The listing builds one solid part. Answer for the finished solid, in the listing's coordinates (mm). A direction names the side the tool comes from. Round coordinates to 2 decimals unless told otherwise and drop trailing zeros. Loops run counter-clockwise (first coordinate to the right, second up) from the corner with the lowest first, then second, coordinate; pieces in that order, holes last. Notation, with made-up numbers: M 60,21 L 107,21 A30 ccw 107,54 Z; hole C 32,17.25 d6. An arc over 180 degrees is marked long. Answer as a JSON object with one key per item and string values.
```python
from build123d import *

# Parameters (mm, degrees)
ESBO_O1_R                  = 19
RESSALTO_EXTRUS_O1_DEPTH   = 7.5
CORTE_EXTRUS_O1_DEPTH      = 28.897132469
CORTE_EXTRUS_O1_DEPTH_BACK = 28.897132469
ESBO_O3_R                  = 13.5
RESSALTO_EXTRUS_O2_DEPTH   = 20
FURO_ROSCADO_DE_M61_D      = 5
FURO_ROSCADO_DE_M51_D      = 4.2
FURO_ROSCADO_DE_M51_DEPTH  = 10
FURO_ROSCADO_DE_M51_TIP    = 1.2618073


with BuildPart() as part:
    # Esboço1 → Ressalto-extrusão1 (new, symmetric)
    with BuildSketch(Plane.XY):
        Circle(ESBO_O1_R)
    extrude(amount=RESSALTO_EXTRUS_O1_DEPTH, both=True)

    # Esboço2 → Corte-extrusão1 (cut, two sides: drawn at the far end of the back side and taken through both)
    with BuildSketch(Plane(origin=(0, 0, 0), x_dir=(1, 0, 0), z_dir=(0, 1, 0)).offset(-CORTE_EXTRUS_O1_DEPTH_BACK)):
        with BuildLine():
            Line((-96.112462059, -41.105261283), (-19, 2.5))
            ThreePointArc((-19, 2.5), (0, 7.5), (19, 2.5))
            Line((19, 2.5), (96.112462059, -41.105261283))
            Line((96.112462059, -41.105261283), (96.112462059, 136.069800352))
            Line((96.112462059, 136.069800352), (-96.112462059, 136.069800352))
            Line((-96.112462059, 136.069800352), (-96.112462059, -41.105261283))
        make_face()
    extrude(amount=CORTE_EXTRUS_O1_DEPTH + CORTE_EXTRUS_O1_DEPTH_BACK, mode=Mode.SUBTRACT)

    # Esboço3 → Ressalto-extrusão2 (add)
    with BuildSketch(Plane.XY.offset(7.5)):
        Circle(ESBO_O3_R)
    extrude(amount=RESSALTO_EXTRUS_O2_DEPTH)

    # Furo roscado de M61 (through all)
    with Locations(Plane.XY.offset(27.5)):
        with Locations((0, 0)):
            Hole(FURO_ROSCADO_DE_M61_D / 2)

    # Furo roscado de M51
    with Locations(Plane(origin=(0, 14, 0), x_dir=(1, 0, 0), z_dir=(0, 1, 0))):
        with Locations((0, -17.5)):
            Hole(FURO_ROSCADO_DE_M51_D / 2, depth=FURO_ROSCADO_DE_M51_DEPTH)
            with Locations((0, 0, -(FURO_ROSCADO_DE_M51_DEPTH + FURO_ROSCADO_DE_M51_TIP / 2))):  # 118° drill point
                Cone(0, FURO_ROSCADO_DE_M51_D / 2, FURO_ROSCADO_DE_M51_TIP, mode=Mode.SUBTRACT)


solid = part.part
```
Item 1: The part is cut by section D-D (x = -7). Give the vertices of the cut face in (y, z).
Values follow:
{"outline": "M -17.66,-6.86 L 17.66,-6.86 L 17.66,7.5 L 11.54,7.5 L 11.54,27.5 L -11.54,27.5 L -11.54,7.5 L -17.66,7.5 Z"}
Item 2: Flat-ended cylindrical pins translate along their axes: P1, Ø6.5, axis at x = 0, z = 17.5, coming from the -Y side; P2, Ø3, axis at x = 0, y = 0, coming from the +Z side; P3, Ø1, axis at y = -5.5, z = 9, coming from the +X side; P4, Ø2, axis at x = 12.5, z = 3.5, coming from the +Y side. Find the tip coordinate at first contact, or state that the pin passes through.
Values follow:
{"P1": "y = -13.5", "P2": "through", "P3": "x = 12.54", "P4": "y = 15.12"}
Item 3: Straight lines are drawn through the part: line 1 (Y direction, x = 0, z = 2); line 2 (Y direction, x = 0, z = 14); line 3 (Z direction, x = 0, y = 8.25). For each, find the intervals that lie inside material, in ascending order.
Values follow:
{"line 1": "-19 to -2.5, 2.5 to 19", "line 2": "-13.5 to -2.5, 2.5 to 13.5", "line 3": "-7.5 to 15.4, 19.6 to 27.5"}
Item 4: Determine the mould class of faces 4 (the face through (0.54, -2.44, 9.75)), 5 (the face through (3, 0, 27.5)), 6 (the face through (-2.93, -13.18, 17.36)), 7 (the face through (0.2, 2.96, 17.19)) for opening direction X: released by +X, released by -X, zero draft, split by the parting line, or undercut.
Values follow:
{"face 4": "undercut", "face 5": "zero draft", "face 6": "split by the parting line", "face 7": "undercut"}
Item 5: The part is cut by section C-C (z = 13.5). Give the vertices of the cut face in (x, y).
Values follow:
{"outline": "C 0,0 d27; hole C 0,0 d5"}
Item 6: Which of the six approach directions +Z, -Z, +X, -X, +Y, -Y give full straight-line access (tool end or side, diameter ignored) to faces 1 (the face through (8.767, -16.856, 1.77)), 2 (the face through (-4.5, 12.9, 7.5)), 3 (the face through (0.273, 8.686, 15.418))?
Values follow:
{"face 1": "+Z, -Z", "face 2": "+Z", "face 3": "+Y"}
Item 7: The part is cut by section A-A (y = 11.5). Give the vertices of the cut face in (x, z).
Values follow:
{"outline": "M -15.12,-4.41 A38.6 ccw 15.12,-4.41 L 15.12,7.5 L 7.07,7.5 L 7.07,27.5 L -7.07,27.5 L -7.07,7.5 L -15.12,7.5 Z; hole C 0,17.5 d4.2"}
Item 8: The part is cut by section B-B (y = 0). Give the vertices of the cut face in (x, z).
Values follow:
{"outline": "M -19,-2.5 A38.6 ccw -2.5,-7.42 L -2.5,27.5 L -13.5,27.5 L -13.5,7.5 L -19,7.5 Z; M 2.5,-7.42 A38.6 ccw 19,-2.5 L 19,7.5 L 13.5,7.5 L 13.5,27.5 L 2.5,27.5 Z"}
